Drawing for the job (mm, zero at the part's lowest x, y, z). A direction names the side the tool comes from. Give positions to 0.01 mm unless a question says otherwise; leave off trailing zeros. Order: outer loops, then holes, each group sorted by start corner. A loop starts at its lowest first (then second) coordinate and runs counter-clockwise, first axis right, second up. Notation, with made-up numbers: (-27, 60.5) -> (-17, 60.5) arc R9 cw to (-17, 73.5) -> close; hole circle Ø10 at (13, 14). An arc over 180 degrees is marked (long way). Use one line per item in the form item = value. Start each with the question number.
1) Cut at D-D, the plane x = 18.3. Give the cut face in (y, z).
2) Cut at A-A, the plane y = 40.3. Give the cut face in (x, z), and give its area (3 significant figures).
3) Cut at C-C, the plane z = 5. Give the cut face in (x, y).
4) Drop flat-ended pins along their axis: P1, Ø4, axis at x = 27, z = 2, coming from the +Y side; P2, Ø8.5, axis at x = 62.3, y = 40.3, coming from the +Z side; P3, Ø4, axis at x = 40.3, y = 62.3, coming from the +Z side; P4, Ø5, axis at y = 37, z = 5, coming from the +X side. Give the stop position or say it passes through.
5) Probe line 1 (Y direction, x = 40.3, z = 3); line 2 (Y direction, x = 40.3, z = 5.4); line 3 (Y direction, x = 54.5, z = 3.25). List the from-to ranges inside material, lowest first.
6) Mould opens along Y. For the marked faces 4, 5 and 6 say: pulls with the +Y half, pulls with the -Y half, needs draft (parallel to the pull), parting line crosses it, or undercut.
7) Tool access for the marked faces 1, 2 and 3: list every direction of +Z, -Z, +X, -X, +Y, -Y with a clear straight run to the whole face (end or side of a thin tool).
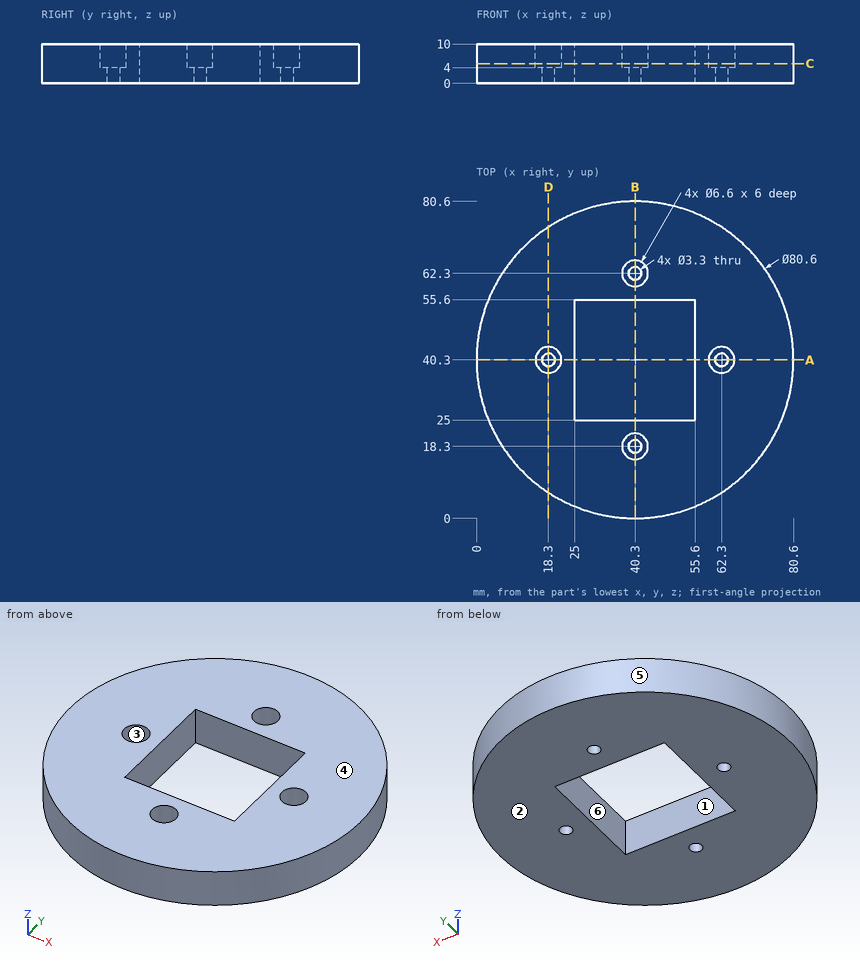
Result:
q1.outline = (6.53, 0) -> (38.65, 0) -> (38.65, 4) -> (37, 4) -> (37, 10) -> (6.53, 10) -> close; (41.95, 0) -> (74.07, 0) -> (74.07, 10) -> (43.6, 10) -> (43.6, 4) -> (41.95, 4) -> close
q2.outline = (0, 0) -> (16.65, 0) -> (16.65, 4) -> (15, 4) -> (15, 10) -> (0, 10) -> close; (19.95, 0) -> (25, 0) -> (25, 10) -> (21.6, 10) -> (21.6, 4) -> (19.95, 4) -> close; (55.6, 0) -> (60.65, 0) -> (60.65, 4) -> (59, 4) -> (59, 10) -> (55.6, 10) -> close; (63.95, 0) -> (80.6, 0) -> (80.6, 10) -> (65.6, 10) -> (65.6, 4) -> (63.95, 4) -> close
q2.area = 394 mm²
q3.outline = circle Ø80.6 at (40.3, 40.3); hole circle Ø6.6 at (18.3, 40.3); hole (25, 25) -> (55.6, 25) -> (55.6, 55.6) -> (25, 55.6) -> close; hole circle Ø6.6 at (40.3, 18.3); hole circle Ø6.6 at (40.3, 62.3); hole circle Ø6.6 at (62.3, 40.3)
q4.P1 = 78.98
q4.P2 = 10
q4.P3 = 4
q4.P4 = 80.59
q5.line_1 = 0 to 16.65, 19.95 to 25, 55.6 to 60.65, 63.95 to 80.6
q5.line_2 = 0 to 15, 21.6 to 25, 55.6 to 59, 65.6 to 80.6
q5.line_3 = 2.58 to 25, 55.6 to 78.02
q6.face_4 = needs draft
q6.face_5 = parting line crosses it
q6.face_6 = undercut
q7.face_1 = +Z, -Z
q7.face_2 = -Z, +X, -X, +Y, -Y
q7.face_3 = +Z
